from build123d import *

# Parameters (mm, degrees)
SKETCH_1_R      = 2.25
SKETCH_1_R_2    = 1.7
SKETCH_1_R_3    = 1.5
EXTRUDE_1_DEPTH = 1.5


with BuildPart() as part:
    # 草图1 → 凸台-拉伸1 (new body)
    with BuildSketch(Plane(origin=(0, 0, 0), x_dir=(1, 0, 0), z_dir=(0, 1, 0))):
        with BuildLine():
            Line((19.75, 2.165063509), (5.096488448, 10.625272348))
            ThreePointArc((5.096488448, 10.625272348), (4.922427124, 10.704637858), (4.736437674, 10.749405626))
            Line((4.736437674, 10.749405626), (-2.101908222, 11.7159388))
            ThreePointArc((-2.101908222, 11.7159388), (-4.61878361, 14.995906411), (-6.744553684, 11.449929699))
            ThreePointArc((-6.744553684, 11.449929699), (-6.675732942, 10.813623622), (-7.006838923, 10.265909693))
            Line((-7.006838923, 10.265909693), (-14.905573539, 3.595069524))
            ThreePointArc((-14.905573539, 3.595069524), (-15.456234647, 3.363542696), (-16.040639512, 3.487249128))
            ThreePointArc((-16.040639512, 3.487249128), (-22, 0), (-16.040639512, -3.487249128))
            ThreePointArc((-16.040639512, -3.487249128), (-15.456234647, -3.363542696), (-14.905573539, -3.595069524))
            Line((-14.905573539, -3.595069524), (-7.006838923, -10.265909693))
            ThreePointArc((-7.006838923, -10.265909693), (-6.675732942, -10.813623622), (-6.744553684, -11.449929699))
            ThreePointArc((-6.744553684, -11.449929699), (-4.61878361, -14.995906411), (-2.101908222, -11.7159388))
            Line((-2.101908222, -11.7159388), (4.736437674, -10.749405626))
            ThreePointArc((4.736437674, -10.749405626), (4.922427124, -10.704637858), (5.096488448, -10.625272348))
            Line((5.096488448, -10.625272348), (19.75, -2.165063509))
            ThreePointArc((19.75, -2.165063509), (20.25, -2.031088913), (20.75, -2.165063509))
            ThreePointArc((20.75, -2.165063509), (24.5, 0), (20.75, 2.165063509))
            ThreePointArc((20.75, 2.165063509), (20.25, 2.031088913), (19.75, 2.165063509))
        make_face()
        Circle(SKETCH_1_R, mode=Mode.SUBTRACT)
        with Locations((-18, 0)):
            Circle(SKETCH_1_R_2, mode=Mode.SUBTRACT)
        with Locations((22, 0)):
            Circle(SKETCH_1_R_3, mode=Mode.SUBTRACT)
        with Locations((-4.47577596, 12.5)):
            Circle(SKETCH_1_R_3, mode=Mode.SUBTRACT)
        with Locations((-4.47577596, -12.5)):
            Circle(SKETCH_1_R_3, mode=Mode.SUBTRACT)
        with BuildLine():
            Line((2.23143448, 9.588554578), (-1.256530939, 10.081544307))
            ThreePointArc((-1.256530939, 10.081544307), (-2.171731289, 9.72303877), (-2.33794765, 8.754281823))
            Line((-2.33794765, 8.754281823), (-0.872808817, 4.662424773))
            ThreePointArc((-0.872808817, 4.662424773), (-0.512657064, 4.185850496), (0.054926934, 3.999622861))
            ThreePointArc((0.054926934, 3.999622861), (0.187612888, 3.995597753), (0.320092213, 3.987172052))
            ThreePointArc((0.320092213, 3.987172052), (0.902629068, 4.119395878), (1.305852753, 4.56012594))
            Line((1.305852753, 4.56012594), (2.997222742, 8.174556771))
            ThreePointArc((2.997222742, 8.174556771), (2.970810351, 9.074617878), (2.23143448, 9.588554578))
        make_face(mode=Mode.SUBTRACT)
        with BuildLine():
            Line((19, 0.866025404), (5.956182941, 8.396876694))
            ThreePointArc((5.956182941, 8.396876694), (5.156119776, 8.484770625), (4.550445454, 7.954690416))
            Line((4.550445454, 7.954690416), (2.664458984, 3.924367251))
            ThreePointArc((2.664458984, 3.924367251), (2.584431714, 3.332397688), (2.856157177, 2.800422501))
            ThreePointArc((2.856157177, 2.800422501), (4, 0), (2.856157177, -2.800422501))
            ThreePointArc((2.856157177, -2.800422501), (2.584431714, -3.332397688), (2.664458984, -3.924367251))
            Line((2.664458984, -3.924367251), (4.550445454, -7.954690416))
            ThreePointArc((4.550445454, -7.954690416), (5.156119776, -8.484770625), (5.956182941, -8.396876694))
            Line((5.956182941, -8.396876694), (19, -0.866025404))
            ThreePointArc((19, -0.866025404), (19.5, 0), (19, 0.866025404))
        make_face(mode=Mode.SUBTRACT)
        with BuildLine():
            Line((-2.33794765, -8.754281823), (-0.872808817, -4.662424773))
            ThreePointArc((-0.872808817, -4.662424773), (-0.512657064, -4.185850496), (0.054926934, -3.999622861))
            ThreePointArc((0.054926934, -3.999622861), (0.187612888, -3.995597753), (0.320092213, -3.987172052))
            ThreePointArc((0.320092213, -3.987172052), (0.902629068, -4.119395878), (1.305852753, -4.56012594))
            Line((1.305852753, -4.56012594), (2.997222742, -8.174556771))
            ThreePointArc((2.997222742, -8.174556771), (2.970810351, -9.074617878), (2.23143448, -9.588554578))
            Line((2.23143448, -9.588554578), (-1.256530939, -10.081544307))
            ThreePointArc((-1.256530939, -10.081544307), (-2.171731289, -9.72303877), (-2.33794765, -8.754281823))
        make_face(mode=Mode.SUBTRACT)
        with BuildLine():
            Line((-5.622052564, 9.472053038), (-13.937734763, 2.449081695))
            ThreePointArc((-13.937734763, 2.449081695), (-14.258158429, 1.944937864), (-14.23400713, 1.348071847))
            ThreePointArc((-14.23400713, 1.348071847), (-14, 0), (-14.23400713, -1.348071847))
            ThreePointArc((-14.23400713, -1.348071847), (-14.258158429, -1.944937864), (-13.937734763, -2.449081695))
            Line((-13.937734763, -2.449081695), (-5.622052564, -9.472053038))
            ThreePointArc((-5.622052564, -9.472053038), (-4.717022681, -9.673722513), (-4.035359228, -9.045164955))
            Line((-4.035359228, -9.045164955), (-2.285010045, -4.156769069))
            ThreePointArc((-2.285010045, -4.156769069), (-2.260804326, -3.559905256), (-2.581182025, -3.055732213))
            ThreePointArc((-2.581182025, -3.055732213), (-4, 0), (-2.581182025, 3.055732213))
            ThreePointArc((-2.581182025, 3.055732213), (-2.260804326, 3.559905256), (-2.285010045, 4.156769069))
            Line((-2.285010045, 4.156769069), (-4.035359228, 9.045164955))
            ThreePointArc((-4.035359228, 9.045164955), (-4.717022681, 9.673722513), (-5.622052564, 9.472053038))
        make_face(mode=Mode.SUBTRACT)
    extrude(amount=EXTRUDE_1_DEPTH)


solid = part.part
Verification items for the finished model (mm, model axes). A direction names the side the tool comes from. Coordinates: 2 decimals unless noted, no trailing zeros. Loops run counter-clockwise (first coordinate to the right, second up) from the corner with the lowest first, then second, coordinate; pieces in that order, holes last. Notation, with made-up numbers: (40, 4) -> (76, 4) arc R20 ccw to (76, 17) -> close; hole circle Ø6 at (9, 36). An arc over 180 degrees is marked (long way). Answer as a JSON object with one key per item and string values. Group by question number.
Item 1: Depth check by flat-ended pin: pin 1 (1 mm diameter, centred on x = 16, z = -6, fed in from -Y). Enter the tip coordinate at first touch or a pass-through.
Item 2: Sectioned sample at C-C on z = -12.5. Record the boundary of the cut face in (x, y).
Item 3: Mould release check, pull along X, two halves, no side actions. Record for faces 1 (the cylindrical face through (-4.7, 0.74, -9.67)), 2 (the cylindrical face through (-6.68, 0.74, 10.8)): +X half, -X half, draft (parallel to the pull), parting line (faces both ways), or undercut.
Item 4: Sectioned sample at B-B on z = 0. Record the boundary of the cut face in (x, y).
Item 5: Scan lines: probe 1 along Z at (x, y) = (22, 1.2); probe 2 along Z at (x, y) = (0, 0.7); probe 3 along X at (y, z) = (0.6, -12.5). Record each from-to range of solid material in increasing order.
Item 6: Sectioned sample at D-D on z = -7. Record the boundary of the cut face in (x, y).
Item 7: Sectioned sample at A-A on x = -18. Record the boundary of the cut face in (y, z), plus the area to 3 significant figures.
Item 8: Tool access check on faces 3 (the cylindrical face through (-0.52, 0.74, -4.19)), 4 (the cylindrical face through (-15.448, 0.74, -3.364)). Record the directions out of +Z, -Z, +X, -X, +Y, -Y that give a thin tool (end or side, any length) a straight path to the whole face; none if there is none.
Evaluation:
{
 "1": {"pin 1": "passes through"},
 "2": {"outline": "(-6.98, 0) -> (-5.98, 0) -> (-5.98, 1.5) -> (-6.98, 1.5) -> close; (-2.98, 0) -> (-1.98, 0) -> (-1.98, 1.5) -> (-2.98, 1.5) -> close"},
 "3": {"face 1": "undercut", "face 2": "-X half"},
 "4": {"outline": "(-22, 0) -> (-19.7, 0) -> (-19.7, 1.5) -> (-22, 1.5) -> close; (-16.3, 0) -> (-14, 0) -> (-14, 1.5) -> (-16.3, 1.5) -> close; (-4, 0) -> (-2.25, 0) -> (-2.25, 1.5) -> (-4, 1.5) -> close; (2.25, 0) -> (4, 0) -> (4, 1.5) -> (2.25, 1.5) -> close; (19.5, 0) -> (20.5, 0) -> (20.5, 1.5) -> (19.5, 1.5) -> close; (23.5, 0) -> (24.5, 0) -> (24.5, 1.5) -> (23.5, 1.5) -> close"},
 "5": {"probe 1": "z = -2.5 to -1.5, 1.5 to 2.5", "probe 2": "z = -11.42 to -9.9, -4 to -2.25, 2.25 to 4, 9.9 to 11.42", "probe 3": "x = -6.98 to -5.98, -2.98 to -1.98"},
 "6": {"outline": "(-10.87, 0) -> (-8.55, 0) -> (-8.55, 1.5) -> (-10.87, 1.5) -> close; (-3.3, 0) -> (-1.71, 0) -> (-1.71, 1.5) -> (-3.3, 1.5) -> close; (2.45, 0) -> (4.1, 0) -> (4.1, 1.5) -> (2.45, 1.5) -> close; (8.38, 0) -> (11.38, 0) -> (11.38, 1.5) -> (8.38, 1.5) -> close"},
 "7": {"outline": "(0, -4) -> (1.5, -4) -> (1.5, -1.7) -> (0, -1.7) -> close; (0, 1.7) -> (1.5, 1.7) -> (1.5, 4) -> (0, 4) -> close", "area": "6.90 mm²"},
 "8": {"face 3": "+Y, -Y", "face 4": "-Z, +Y, -Y"}
}
